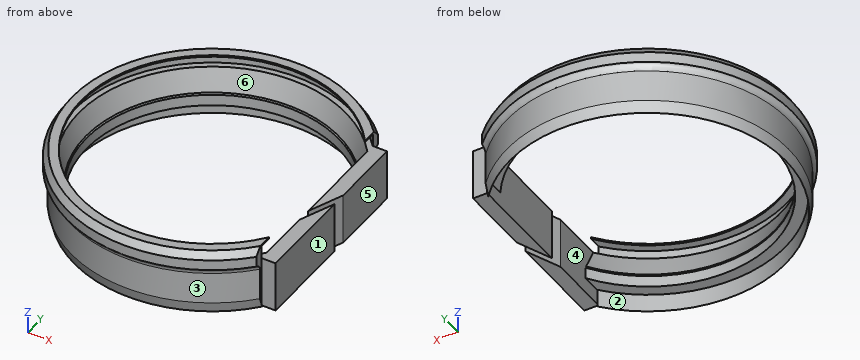
```python
from build123d import *

# Parameters (mm, degrees)
F0_W      = 1.4
F0_H      = 0.3
F0_W_2    = 2
F0_H_2    = 2
F4_SIZE2  = 0.49999
F4_SIZE   = 1.99999
F5_R      = 0.5
F7_DEPTH  = 25
F9_DEPTH  = 9
F11_DEPTH = 100


# Not quite as in the source:
# - a fillet or chamfer that OpenCascade refuses, or shapes differently, is made with other operations: its cross-section is extruded or revolved along the edge and cut away or added
# - a fillet or chamfer is up to 0.001 mm smaller than in the source, because OpenCascade refuses the exact size


with BuildPart() as f1:
    # F0 (on Front) → F1 (revolve)
    with BuildSketch(Plane.XZ):
        Polygon((-24.5, 0), (-25.5, 0), (-25.5, -3.1555826106), (-24.8, -3.1555826106), (-24.8, -11.9555826106), (-24.3, -11.9555826106), (-24.3, -4.9555826106), (-23.391673381, -4.9555826106), (-22.9283481642, -6.5), (-22.3, -6.5), (-23.5, -2.5), (-24.5, -2.5), (-24.5, -0.3), align=None)
        with Locations((-23.8, -0.15)):
            Rectangle(F0_W, F0_H)
    revolve(axis=Axis((0, 0, 1.0689813644), (0, 0, -1)))

    # F2: chamfer of 0.8 x 1.3 on 1 edges, made by hand

    # F2_s1 → F2_t2 (revolve, cut)
    with BuildSketch(Plane.XZ):
        Polygon((-25.5, -1.3), (-24.7, 0), (-25.5, 0), align=None)
    revolve(axis=Axis((0, 0, 0), (0, 0, -1)), mode=Mode.SUBTRACT)

    # F3: fillet of radius 1.4 on 1 edges, made by hand

    # F3_s1 → F3_t2 (revolve)
    with BuildSketch(Plane.XZ):
        with BuildLine():
            ThreePointArc((-25.4997998621, -3.1552362801), (-24.9872079854, -3.6681342757), (-24.7996, -4.3685755865))
            Line((-24.7996, -4.3685755865), (-24.6594634315, -4.3685755865))
            ThreePointArc((-24.6594634315, -4.3685755865), (-24.6598634315, -3.7620790985), (-24.6598634315, -3.1555826106))
            Line((-24.6598634315, -3.1555826106), (-24.8, -3.015446042))
            ThreePointArc((-24.8, -3.015446042), (-25.1498999311, -3.015446042), (-25.4296832798, -3.0339023494))
            Line((-25.4296832798, -3.0339023494), (-25.4997998621, -3.1552362801))
        make_face()
    revolve(axis=Axis((0, 0, -3.1555826106), (0, 0, -1)))

    # F4 (size 2 and 0.5 in the source; OpenCascade refuses exactly that, so slightly less here)
    f4_edges = [f1.edges().sort_by_distance(p)[0] for p in [
        (24.8, 0, -11.955583),
    ]]
    chamfer(f4_edges, length=F4_SIZE, length2=F4_SIZE2)

    # F5
    f5_edges = [f1.edges().sort_by_distance(p)[0] for p in [
        (23.391673, 0, -4.955583),
    ]]
    fillet(f5_edges, radius=F5_R)


with BuildPart() as f1b:
    # F0 (on Front) → F1, piece 2 (revolve)
    with BuildSketch(Plane.XZ):
        with Locations((-23.2, -7.8631715626)):
            Rectangle(F0_W_2, F0_H_2)
    revolve(axis=Axis((0, 0, 1.0689813644), (0, 0, -1)))


with BuildPart() as f7_tool:
    # F6 (on Top) → F7 (new body)
    with BuildSketch(Plane.XY):
        Polygon((18.4932420089, 17.5570498661), (18.4932420089, 14.5), (18.4932420089, -14.5), (18.4932420089, -17.5570498661), (23.4932420089, -17.5570498661), (23.4932420089, 17.5570498661), align=None)
        Polygon((18.4932420089, 29.2936375588), (18.4932420089, 17.5570498661), (23.4932420089, 17.5570498661), (23.4932420089, -17.5570498661), (18.4932420089, -17.5570498661), (18.4932420089, -27.3348336816), (60.3667099652, -27.3348336816), (60.3667099652, 29.2936375588), align=None)
    extrude(amount=-F7_DEPTH)


with BuildPart() as f1_1:
    add(f1.part)

    # F7: cut by f7_tool
    add(f7_tool.part, mode=Mode.SUBTRACT)



with BuildPart() as f1b_1:
    add(f1b.part)

    # F7: cut by f7_tool
    add(f7_tool.part, mode=Mode.SUBTRACT)


with BuildPart() as f1_2:
    add(f1_1.part)

    add(f1b_1.part)  # F9 merges F1b
    # F8 (on face) → F9 (join)
    with BuildSketch(Plane.XY.offset(-2.5)):
        Polygon((20.9932420089, 16.07015868), (18.4932420089, 16.07015868), (18.4932420089, 14.5), (18.4932420089, -14.5), (18.4932420089, -16.07015868), (20.9932420089, -16.07015868), align=None)
    extrude(amount=-F9_DEPTH)

    # F10 (on Top) → F11 (cut)
    with BuildSketch(Plane.XY):
        Polygon((28.4932420089, 21.42984132), (15.9932420089, -8.57015868), (15.9932420089, -11.07015868), (28.4932420089, 18.92984132), align=None)
    extrude(amount=-F11_DEPTH, mode=Mode.SUBTRACT)


solid = f1_2.part
```
Here's how the part is built. I have some questions about the finished solid (model axes, mm). Face numbers are marked on the shaded views. A direction names the side the tool comes from. Give positions to 0.01 mm unless a question says otherwise; leave off trailing zeros. Use one line per item in the form item = value. Start each with the question number.
1) Please list where these lines run through material, in increasing order: line 1 along Y through (x, z) = (0, -1.85); line 2 along Y through (x, z) = (0, -0.15); line 3 along X through (y, z) = (-9, -6.25).
2) For P1, Ø5, axis at x = -6, z = -5.5, coming from the +Y side; P2, Ø3, axis at x = 12, z = -2, coming from the +Y side; P3, Ø0.8, axis at x = 20.5, y = 8, coming from the -Z side; P4, Ø22.5, axis at x = 9.5, y = 8.5, coming from the +Z side, each with a flat end and sliding along its axis, tell me the tip position at first contact or that it passes through.
3) Thinking about a two-plate mould opening in X: for the marked faces 3, 4, 5 and 6, which applies, +X half, -X half, draft (parallel to the pull), parting line (faces both ways), or undercut?
4) Which directions (+Z, -Z, +X, -X, +Y, -Y) give clear straight access to the entire face, cutting with the end or side of a thin tool? Please do the marked faces 1 and 2.
5) Imagine slicing it at C-C (x = 17). Count the separate pieces of the cut face and the enclosed holes in it, then the cut area to 3 significant figures.
Check values:
q1.line_1 = -25.5 to -24.5, 24.5 to 25.5
q1.line_2 = -24.79 to -23.1, 23.1 to 24.79
q1.line_3 = -23.11 to -22.57, -21.17 to -20.49, 18.49 to 20.99
q2.P1 = 24.98
q2.P2 = 23.24
q2.P3 = -11.5
q2.P4 = 0
q3.face_3 = parting line
q3.face_4 = undercut
q3.face_5 = +X half
q3.face_6 = undercut
q4.face_1 = +Z, -Z, +X, +Y, -Y
q4.face_2 = -Z
q5.separate_pieces = 4
q5.enclosed_holes = 0
q5.area = 43.3 mm^2
